```python
from build123d import *

# Parameters (mm, degrees)
SKETCH1_R           = 1.5
SKETCH1_R_2         = 1.4
BOSS_EXTRUDE1_DEPTH = 4
SKETCH2_R           = 1.4
CUT_EXTRUDE1_DEPTH  = 10


with BuildPart() as part:
    # Sketch1 → Boss-Extrude1 (new body)
    with BuildSketch(Plane.XY):
        with BuildLine():
            Line((-10, 0), (-7.652901889, -30))
            ThreePointArc((-7.652901889, -30), (0, -37.652901889), (7.652901889, -30))
            Line((7.652901889, -30), (10, 0))
            ThreePointArc((10, 0), (0, 10), (-10, 0))
        make_face()
        Circle(SKETCH1_R, mode=Mode.SUBTRACT)
        with Locations((7, 0)):
            Circle(SKETCH1_R_2, mode=Mode.SUBTRACT)
        with Locations((0, -7)):
            Circle(SKETCH1_R_2, mode=Mode.SUBTRACT)
        with Locations((-7, 0)):
            Circle(SKETCH1_R_2, mode=Mode.SUBTRACT)
        with Locations((0, 7)):
            Circle(SKETCH1_R_2, mode=Mode.SUBTRACT)
        with Locations((0, -30)):
            Circle(SKETCH1_R_2, mode=Mode.SUBTRACT)
    extrude(amount=BOSS_EXTRUDE1_DEPTH)

    # Sketch2 → Cut-Extrude1 (cut)
    with BuildSketch(Plane.XY.offset(4)):
        with BuildLine():
            ThreePointArc((9.878325443, -1.55521267), (0, -10), (-9.878325443, -1.55521267))
            Line((-9.878325443, -1.55521267), (-7.652901889, -30))
            ThreePointArc((-7.652901889, -30), (0, -37.652901889), (7.652901889, -30))
            Line((7.652901889, -30), (9.878325443, -1.55521267))
        make_face()
        with Locations((0, -30)):
            Circle(SKETCH2_R, mode=Mode.SUBTRACT)
    extrude(amount=-CUT_EXTRUDE1_DEPTH, mode=Mode.SUBTRACT)


solid = part.part
```
For this review, take the finished solid that the model builds, in its own axes (mm). Give positions to 0.01 mm unless a question says otherwise; leave off trailing zeros. Write each loop counter-clockwise with the first axis right and the second up, starting at its lowest first coordinate (ties: lowest second). Pieces come first, ordered by that corner, then holes. Notation, with made-up numbers: M 55,28.25 L 107,28.25 A20 ccw 107,66.25 Z; hole C -35.5,49 d6. An arc over 180 degrees is marked long. Answer as a JSON object with one key per item and string values. Group by question number.
Item 1: Consider section A-A on x = -7.25. Write out the cut boundary in (y, z).
Item 2: Consider section D-D on y = 1.75. Write out the cut boundary in (x, z), plus the area to 3 significant figures.
Item 3: For probe 1 along Y at (x, z) = (0, 2.35); probe 2 along Y at (x, z) = (7, 3.1); probe 3 along X at (y, z) = (-1, 3.25), list the stretches that pass through material, from the lowest coordinate up. Write a range as [from, to].
Item 4: Consider section B-B on z = 3.45. Write out the cut boundary in (x, y), plus the area to 3 significant figures.
Item 5: Consider section C-C on y = -7. Write out the cut boundary in (x, z), plus the area to 3 significant figures.
Item 6: Draft analysis for pull direction Y (two halves, no side actions). For faces 1 (the cylindrical face through (0, -10, 2)), 2 (the flat face through (0, -2, 0)), 3 (the cylindrical face through (-8.4, 0.06, 1.97)), state which applies: +Y half, -Y half, draft (parallel to the pull), parting line (faces both ways), or undercut.
Item 7: For pin 1 Ø2 at (x, y) = (7, 0) entering from +Z; pin 2 Ø1.5 at (y, z) = (-3.5, 3) entering from +X, all flat-tipped, find the tip position at first contact; note any pin that passes through.
Check result:
{
 "1": {"outline": "M -6.89,0 L -1.38,0 L -1.38,4 L -6.89,4 Z; M 1.38,0 L 6.89,0 L 6.89,4 L 1.38,4 Z"},
 "2": {"outline": "M -9.85,0 L 9.85,0 L 9.85,4 L -9.85,4 Z", "area": "78.8 mm^2"},
 "3": {"probe 1": "y = [-10, -8.4], [-5.6, -1.5], [1.5, 5.6], [8.4, 10]", "probe 2": "y = [-7.14, -1.4], [1.4, 7.14]", "probe 3": "x = [-9.92, -7.98], [-6.02, -1.12], [1.12, 6.02], [7.98, 9.92]"},
 "4": {"outline": "M -10,0 L -9.88,-1.56 A10 ccw 9.88,-1.56 L 10,0 A10 ccw Z; hole C -7,0 d2.8; hole C 0,0 d3; hole C 0,-7 d2.8; hole C 0,7 d2.8; hole C 7,0 d2.8", "area": "282 mm^2"},
 "5": {"outline": "M -7.14,0 L -1.4,0 L -1.4,4 L -7.14,4 Z; M 1.4,0 L 7.14,0 L 7.14,4 L 1.4,4 Z", "area": "45.9 mm^2"},
 "6": {"face 1": "-Y half", "face 2": "draft", "face 3": "undercut"},
 "7": {"pin 1": "passes through", "pin 2": "stops at x = 9.61"}
}
